Can you work these out from the model? Positions are in its coordinate system, mm. Face numbers are marked on the shaded views. A direction names the side the tool comes from. Round coordinates to 2 decimals unless told otherwise and drop trailing zeros. Order: outer loops, then holes, each group sorted by start corner. A loop starts at its lowest first (then second) coordinate and runs counter-clockwise, first axis right, second up. Notation, with made-up numbers: (64.5, -37) -> (115.5, -37) arc R14 ccw to (115.5, -19) -> close; hole circle Ø7 at (47.25, 23.5). An arc over 180 degrees is marked (long way). Use a Markdown table: item, result. Add a question column.
Q1. We'd pull the mould along Z, two halves only. Please class the marked faces 4, 5, 6 and 7: +Z half, -Z half, draft (parallel to the pull), parting line (faces both ways), or undercut.
Q2. If we section it at B-B on x = 27: List the corners of the cut face in (y, z) for me, plus the area to 3 significant figures.
Q3. I need wall thicknesses on line 1 along Y through (x, z) = (13, 34); line 2 along X through (y, z) = (33, 19); line 3 along X through (y, z) = (15.5, 30). Which ranges of each line are inside material? Lowest first, please. Write a range as [from, to].
Q4. I'm going to push flat-ended pins straight in: pin 1 Ø6.5 at (y, z) = (20.5, 44) entering from +X; pin 2 Ø4 at (y, z) = (32.5, 48.5) entering from +X; pin 3 Ø6.5 at (y, z) = (33.5, 28.5) entering from +X. Where does each tip first touch, or does it pass through?
Q5. If we section it at A-A on z = 49: List the corners of the cut face in (x, y) for me.
Q6. For the marked faces 1, 2 and 3, which set-ups out of +Z, -Z, +X, -X, +Y, -Y let a thin tool reach every point of the face, with its end or its side?
Q7. If we section it at D-D on z = 20: List the corners of the cut face in (x, y) for me.
Q8. If we section it at C-C on y = 28.5: List the corners of the cut face in (x, z) for me.
Autodesk Inventor part; units mm, degrees
ref_plane "YZ Plane" through (0, 0, 0) normal (1, 0, 0) x (0, 1, 0)
ref_plane "XZ Plane" through (0, 0, 0) normal (0, 1, 0) x (-1, 0, 0)
ref_plane "XY Plane" through (0, 0, 0) normal (0, 0, 1) x (1, 0, 0)
sketch "Sketch1" plane through (0, 0, 0) normal (0, 0, 1) x (1, 0, 0)
  point P0 (0, 0)
sketch "Sketch2" plane through (0, 0, 0) normal (0, 0, 1) x (1, 0, 0)
  line L0 (0, 0) -> (50.8, 0)
  line L1 (50.8, 0) -> (50.8, 12.7)
  line L2 (50.8, 12.7) -> (12.7, 12.7)
  line L3 (12.7, 12.7) -> (12.7, 25.4)
  line L4 (12.7, 25.4) -> (38.1, 25.4)
  line L5 (38.1, 25.4) -> (38.1, 38.1)
  line L6 (38.1, 38.1) -> (0, 38.1)
  line L7 (0, 38.1) -> (0, 0)
extrude "Extrusion1" add sketch "Sketch2" along normal blind 63.5
sketch "Sketch3" plane through (12.7, 12.7, 0) normal (0, 1, 0) x (1, 0, 0)
  line L0 (38.1, -25.4) -> (25.4, -25.4)
  line L1 (25.4, -25.4) -> (25.4, -63.5)
  line L2 (38.1, -63.5) -> (0, -63.5)
  line L3 (25.4, -63.5) -> (38.1, -63.5)
  line L4 (38.1, -63.5) -> (38.1, -25.4)
  point P0 (-12.7, 0)
extrude "Extrusion2" cut sketch "Sketch3" against normal blind 12.7
sketch "Sketch4" plane through (0, 38.1, 0) normal (0, 1, 0) x (1, 0, 0)
  line L0 (38.1, 0) -> (38.1, -63.5)
  line L1 (38.1, -19.05) -> (31.75, -19.05)
  line L2 (31.75, -19.05) -> (31.75, -12.7)
  line L3 (31.75, -12.7) -> (25.4, -12.7)
  line L4 (25.4, -12.7) -> (25.4, -50.8)
  line L5 (25.4, -50.8) -> (31.75, -50.8)
  line L6 (31.75, -50.8) -> (31.75, -44.45)
  line L7 (31.75, -44.45) -> (38.1, -44.45)
  line L8 (38.1, -44.45) -> (38.1, -19.05)
  point P0 (0, 0)
extrude "Extrusion3" cut sketch "Sketch4" against normal blind 12.7
properties part number "P3-7"
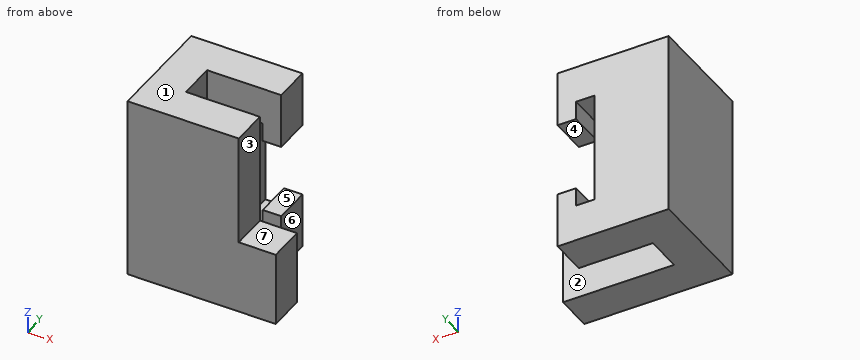
Answer below:
| question | item | result |
|---|---|---|
| 1 | face 4 | undercut |
| 1 | face 5 | undercut |
| 1 | face 6 | draft |
| 1 | face 7 | +Z half |
| 2 | outline | (0, 0) -> (12.7, 0) -> (12.7, 63.5) -> (0, 63.5) -> close; (25.4, 0) -> (38.1, 0) -> (38.1, 12.7) -> (25.4, 12.7) -> close; (25.4, 50.8) -> (38.1, 50.8) -> (38.1, 63.5) -> (25.4, 63.5) -> close |
| 2 | area | 1,130 mm² |
| 3 | line 1 | [0, 12.7], [25.4, 38.1] |
| 3 | line 2 | [0, 25.4], [31.75, 38.1] |
| 3 | line 3 | [0, 12.7] |
| 4 | pin 1 | x = 12.7 |
| 4 | pin 2 | x = 38.1 |
| 4 | pin 3 | x = 25.4 |
| 5 | outline | (0, 0) -> (38.1, 0) -> (38.1, 12.7) -> (12.7, 12.7) -> (12.7, 25.4) -> (25.4, 25.4) -> (25.4, 38.1) -> (0, 38.1) -> close; (31.75, 25.4) -> (38.1, 25.4) -> (38.1, 38.1) -> (31.75, 38.1) -> close |
| 6 | face 1 | +Z, +X, -X, +Y, -Y |
| 6 | face 2 | +Z, -Z, +X |
| 6 | face 3 | +Z, +X, +Y, -Y |
| 7 | outline | (0, 0) -> (50.8, 0) -> (50.8, 12.7) -> (12.7, 12.7) -> (12.7, 25.4) -> (25.4, 25.4) -> (25.4, 38.1) -> (0, 38.1) -> close |
| 8 | outline | (0, 0) -> (38.1, 0) -> (38.1, 19.05) -> (31.75, 19.05) -> (31.75, 12.7) -> (25.4, 12.7) -> (25.4, 50.8) -> (31.75, 50.8) -> (31.75, 44.45) -> (38.1, 44.45) -> (38.1, 63.5) -> (0, 63.5) -> close |
